The listing builds one solid part. Answer for the finished solid, in the listing's coordinates (mm). Give positions to 0.01 mm unless a question says otherwise; leave off trailing zeros. Loops run counter-clockwise (first coordinate to the right, second up) from the corner with the lowest first, then second, coordinate; pieces in that order, holes last.
Item 1: Section A-A, the plane z = 10 is taken. Give the vertices of the cut face in (x, y).
Item 2: Consider line 1 along Y through (x, z) = (-20.5, 7.5); line 2 along Z through (x, y) = (-26, 21); line 3 along Y through (x, z) = (-24, 3). Determine where each line is inside the solid, lowest interval first.
Item 3: Section D-D, the plane y = 33.5 is taken. Give the vertices of the cut face in (x, z).
Item 4: The mould has two halves that part along X. Classify faces 1 (the face through (-12.871, 26, 10)), 2 (the face through (-23, 26, 20)), 3 (the face through (-32.871, 26, 10)), 4 (the face through (-23.76, 26.868, 9.86)): pulls with the +X half, pulls with the -X half, needs draft (parallel to the pull), parting line crosses it, or undercut.
Item 5: Section B-B, the plane x = -25.5 is taken. Give the vertices of the cut face in (y, z), and give its area (3 significant figures).
Item 6: Section C-C, the plane x = -29.5 is taken. Give the vertices of the cut face in (y, z), and give its area (3 significant figures).
from build123d import *

# Parameters (mm, degrees)
SKETCH_W     = 20
SKETCH_H     = 30
SKETCH_R     = 4.1
PAD_DEPTH    = 20
SKETCH001_R  = 4.1
POCKET_DEPTH = 20


with BuildPart() as part:
    # Sketch → Pad (new body)
    with BuildSketch(Plane.XY):
        with Locations((-22.871155, 25.870022)):
            Rectangle(SKETCH_W, SKETCH_H)
        with Locations((-22.871155, 30.870022)):
            Circle(SKETCH_R, mode=Mode.SUBTRACT)
    extrude(amount=PAD_DEPTH)

    # Sketch001 → Pocket (cut)
    with BuildSketch(Plane.YZ.offset(-12.871155)):
        with Locations((20.870022, 10)):
            Circle(SKETCH001_R)
    extrude(amount=-POCKET_DEPTH, mode=Mode.SUBTRACT)


solid = part.part
Worked answers:
1. outline: (-32.87, 10.87) - (-12.87, 10.87) - (-12.87, 16.77) - (-32.87, 16.77) - close; (-32.87, 24.97) - (-12.87, 24.97) - (-12.87, 40.87) - (-32.87, 40.87) - close; hole circle Ø8.2 at (-22.87, 30.87)
2. line 1: y = 10.87 to 17.62, 24.12 to 27.53, 34.21 to 40.87
2. line 2: z = 0 to 5.9, 14.1 to 20
2. line 3: y = 10.87 to 26.93, 34.81 to 40.87
3. outline: (-32.87, 0) - (-26.02, 0) - (-26.02, 20) - (-32.87, 20) - close; (-19.73, 0) - (-12.87, 0) - (-12.87, 20) - (-19.73, 20) - close
4. face 1: pulls with the +X half
4. face 2: needs draft
4. face 3: pulls with the -X half
4. face 4: undercut
5. outline: (10.87, 0) - (27.72, 0) - (27.72, 20) - (10.87, 20) - close; (34.02, 0) - (40.87, 0) - (40.87, 20) - (34.02, 20) - close; hole circle Ø8.2 at (20.87, 10)
5. area: 421 mm2
6. outline: (10.87, 0) - (40.87, 0) - (40.87, 20) - (10.87, 20) - close; hole circle Ø8.2 at (20.87, 10)
6. area: 547 mm2
